Check sheet for the drawn part. Datum: minimum x, y, z corner. Units: mm. A direction names the side the tool comes from. Coordinates: 2 decimals unless noted, no trailing zeros. Loops run counter-clockwise (first coordinate to the right, second up) from the corner with the lowest first, then second, coordinate; pieces in that order, holes last. Notation, with made-up numbers: (25.25, 46.25) - (30.25, 46.25) arc R10 cw to (30.25, 58.25) - close; hole circle Ø11 at (-17, 34.25). An arc over 180 degrees is marked (long way). Answer as CSV lines item,"result". Start each with the question number.
1. Set-up check for the marked faces 1 and 2: record each of +Z, -Z, +X, -X, +Y, -Y from which the full face is reachable in a straight line by a thin tool's end or side.
2. Cross-section at C-C (y = 5.75). Enter the section's corners in (x, z), plus the area to 3 significant figures.
3. Material ranges on line 1 (Z direction, x = 26, y = 1.75); line 2 (X direction, y = 4, z = 27.5), recorded low to high. Write a range as [from, to].
4. Cross-section at B-B (z = 28.5). Enter the section's corners in (x, y), plus the area to 3 significant figures.
5. Gauge pin test, flat end, axial feed: P1, Ø3, axis at y = 17, z = 4, coming from the +X side. Record the tip position at first contact, or that the pin passes through.
6. Cross-section at D-D (z = 6). Enter the section's corners in (x, y).
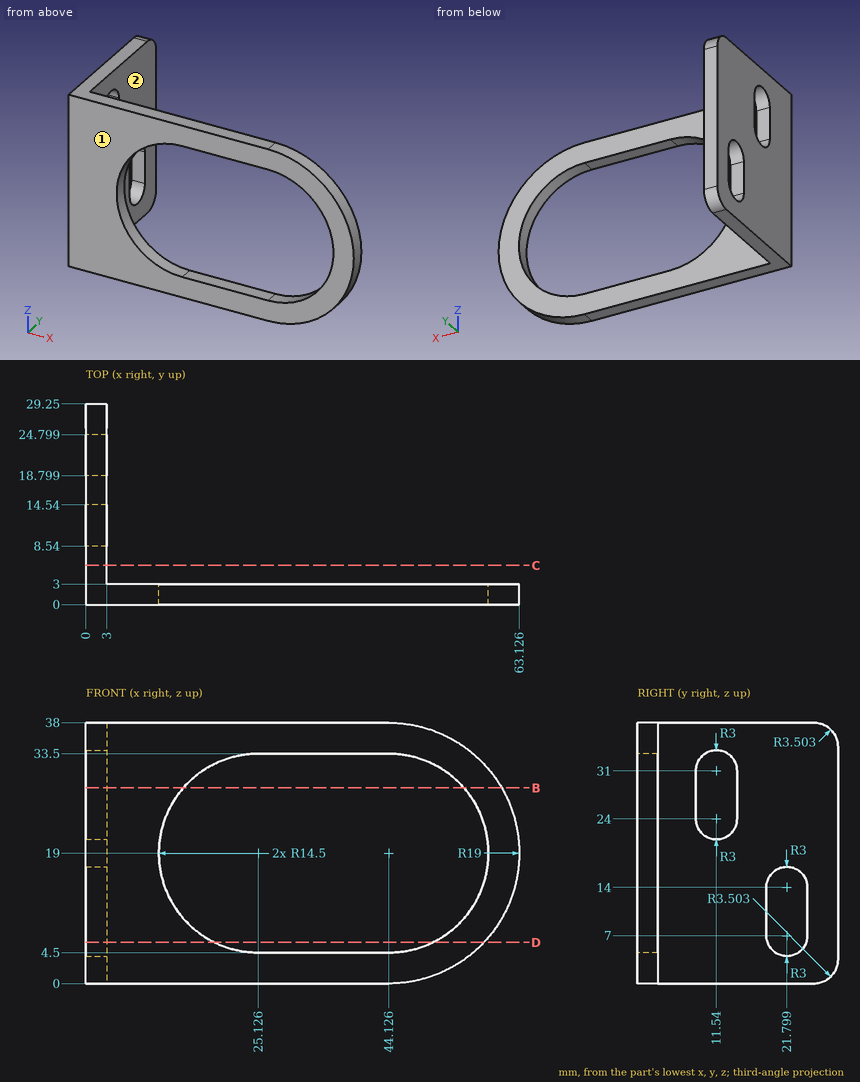
Values follow:
1,face 1,"+Z, -Z, +X, -X, -Y"
1,face 2,"+Z, -Z, +X, +Y"
2,outline,"(0, 0) - (3, 0) - (3, 38) - (0, 38) - close"
2,area,"114 mm²"
3,line 1,"z = [0, 4.5], [33.5, 38]"
3,line 2,"x = [0, 3]"
4,outline,"(0, 0) - (14.17, 0) - (14.17, 3) - (3, 3) - (3, 8.54) - (0, 8.54) - close; (0, 14.54) - (3, 14.54) - (3, 29.25) - (0, 29.25) - close; (55.08, 0) - (60.58, 0) - (60.58, 3) - (55.08, 3) - close"
4,area,"120 mm²"
5,P1,"stops at x = 3"
6,outline,"(0, 0) - (18.7, 0) - (18.7, 3) - (3, 3) - (3, 18.97) - (0, 18.97) - close; (0, 24.63) - (3, 24.63) - (3, 29.25) - (0, 29.25) - close; (50.55, 0) - (57.98, 0) - (57.98, 3) - (50.55, 3) - close"
